from build123d import *

# Parameters (mm, degrees)
ESQUISSE1_W                  = 570
ESQUISSE1_H                  = 150
BOSS_EXTRU_1_DEPTH           = 27
ENL_V_MAT_EXTRU_1_DEPTH      = 591.024575759
ENL_V_MAT_EXTRU_1_DEPTH_BACK = 591.024575759


with BuildPart() as part:
    # Esquisse1 → Boss.-Extru.1 (new body)
    with BuildSketch(Plane.XY):
        with Locations((285, 75)):
            Rectangle(ESQUISSE1_W, ESQUISSE1_H)
    extrude(amount=BOSS_EXTRU_1_DEPTH)

    # Esquisse2 → Enlèv. mat.-Extru.1 (cut, two sides: drawn at the far end of the back side and taken through both)
    with BuildSketch(Plane.XY.offset(27).offset(-ENL_V_MAT_EXTRU_1_DEPTH_BACK)):
        Polygon((75, 0), (570, 75), (570, 0), align=None)
    extrude(amount=ENL_V_MAT_EXTRU_1_DEPTH + ENL_V_MAT_EXTRU_1_DEPTH_BACK, mode=Mode.SUBTRACT)


solid = part.part
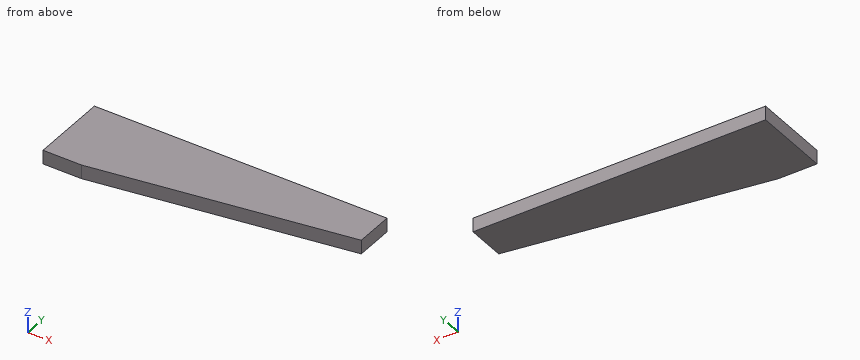
Geometry: final body of the model. Coordinates: model frame, mm. Coordinates: 2 decimals unless noted, no trailing zeros. Loops run counter-clockwise (first coordinate to the right, second up) from the corner with the lowest first, then second, coordinate; pieces in that order, holes last. Notation, with made-up numbers: M 66,25.25 L 124,25.25 A27 ccw 124,50.25 Z; hole C 49,16 d1. An arc over 180 degrees is marked long. One line per item, written item: value. Start each with the question number.
1) Cut plane C-C (x = 438.5). Return loops of the section in (y, z).
2) Cut plane B-B (y = 45). Return loops of the section in (x, z).
3) Pin query (flat end, axial travel): P1, Ø12, axis at y = 76.5, z = 15.5, coming from the -X side; P2, Ø1, axis at x = 477, z = 12.5, coming from the -Y side; P3, Ø4, axis at x = 233, z = 21.5, coming from the -Y side. Return the tip coordinate at first contact, or that it passes through.
4) Material intervals for L1, parallel to Y at x = 218.5, z = 21.5; L2, parallel to Y at x = 330.5, z = 14.5, sorted ascending. Write a range as from..to.
5) Cut plane A-A (z = 6.5). Return loops of the section in (x, y).
Evaluation:
1. outline: M 55.08,0 L 150,0 L 150,27 L 55.08,27 Z
2. outline: M 0,0 L 372,0 L 372,27 L 0,27 Z
3. P1: x = 0
3. P2: y = 60.83
3. P3: y = 23.64
4. L1: 21.74..150
4. L2: 38.71..150
5. outline: M 0,0 L 75,0 L 570,75 L 570,150 L 0,150 Z
